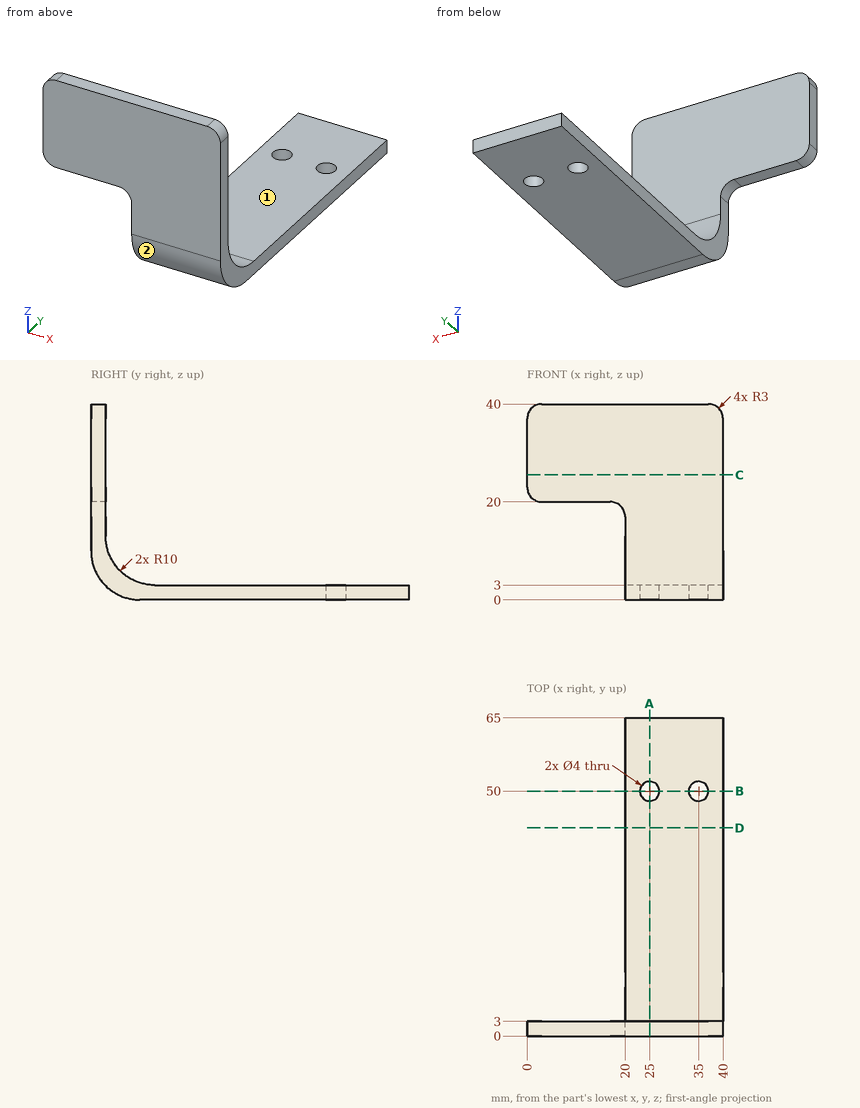
Here's the drawing with two shaded views (mm, measured from the low corner). I have some questions. A direction names the side the tool comes from. Give positions to 0.01 mm unless a question says otherwise; leave off trailing zeros. Loops run counter-clockwise (first coordinate to the right, second up) from the corner with the lowest first, then second, coordinate; pieces in that order, holes last. Notation, with made-up numbers: M -34.75,30 L -15.75,30 A22 cw -15.75,48 Z; hole C 8.5,43.5 d5. An arc over 180 degrees is marked long. Answer in a Markdown table with one row per item.
1. Suppose I cut it at C-C on z = 25.5. Write out the boundary of the cut face in (x, y), plus the area to 3 significant figures.
Taken from the geometry:
| item | result |
|---|---|
| outline | M 0,0 L 40,0 L 40,3 L 0,3 Z |
| area | 120 mm² |
2. Suppose I cut it at D-D on y = 42.5. Write out the boundary of the cut face in (x, z).
Taken from the geometry:
| item | result |
|---|---|
| outline | M 20,0 L 40,0 L 40,3 L 20,3 Z |
3. Suppose I cut it at A-A on x = 25. Write out the boundary of the cut face in (y, z), plus the area to 3 significant figures.
Taken from the geometry:
| item | result |
|---|---|
| outline | M 0,10 A10 ccw 10,0 L 48,0 L 48,3 L 13,3 A10 cw 3,13 L 3,40 L 0,40 Z; M 52,0 L 65,0 L 65,3 L 52,3 Z |
| area | 294 mm² |
4. Which directions (+Z, -Z, +X, -X, +Y, -Y) give clear straight access to the entire face, cutting with the end or side of a thin tool? Please do the marked faces 1 and 2.
Taken from the geometry:
| item | result |
|---|---|
| face 1 | +Z, +X, -X, +Y |
| face 2 | -Z, +X, -X, -Y |
5. If I drill on line 1 along Y through (x, z) = (38, 15.5); line 2 along Y through (x, z) = (25, 1.4), over which ranges is the centre line in solid material (lowest first)?
Taken from the geometry:
| item | result |
|---|---|
| line 1 | y = 0 to 3 |
| line 2 | y = 4.9 to 48, 52 to 65 |
6. For pin 1 Ø1.5 at (x, y) = (26.5, 55) entering from +Z; pin 2 Ø10 at (x, z) = (35.5, 8) entering from -Y; pin 3 Ø1.5 at (x, y) = (8.5, 1) entering from -Z; pin 4 Ø21.5 at (x, z) = (19, 21.5) entering from +Y, each with a flat end and sliding along its axis, tell me the tip position at first contact or that it passes through.
Taken from the geometry:
| item | result |
|---|---|
| pin 1 | stops at z = 3 |
| pin 2 | stops at y = 0 |
| pin 3 | stops at z = 20 |
| pin 4 | stops at y = 3.25 |
7. Suppose I cut it at B-B on y = 50. Write out the boundary of the cut face in (x, z).
Taken from the geometry:
| item | result |
|---|---|
| outline | M 20,0 L 23,0 L 23,3 L 20,3 Z; M 27,0 L 33,0 L 33,3 L 27,3 Z; M 37,0 L 40,0 L 40,3 L 37,3 Z |
